The figure shows three views and two pictorial views of one solid part (mm, origin at its lowest corner). Answer the questions. A direction names the side the tool comes from. Coordinates: 2 decimals unless noted, no trailing zeros. Write each loop counter-clockwise with the first axis right and the second up, starting at its lowest first coordinate (ties: lowest second). Pieces come first, ordered by that corner, then holes. Notation, with made-up numbers: M 67.5,53.5 L 92.5,53.5 A12 ccw 92.5,71.5 Z; hole C 26.25,8 d11. An arc over 180 degrees is marked long. Write item = value, one per line.
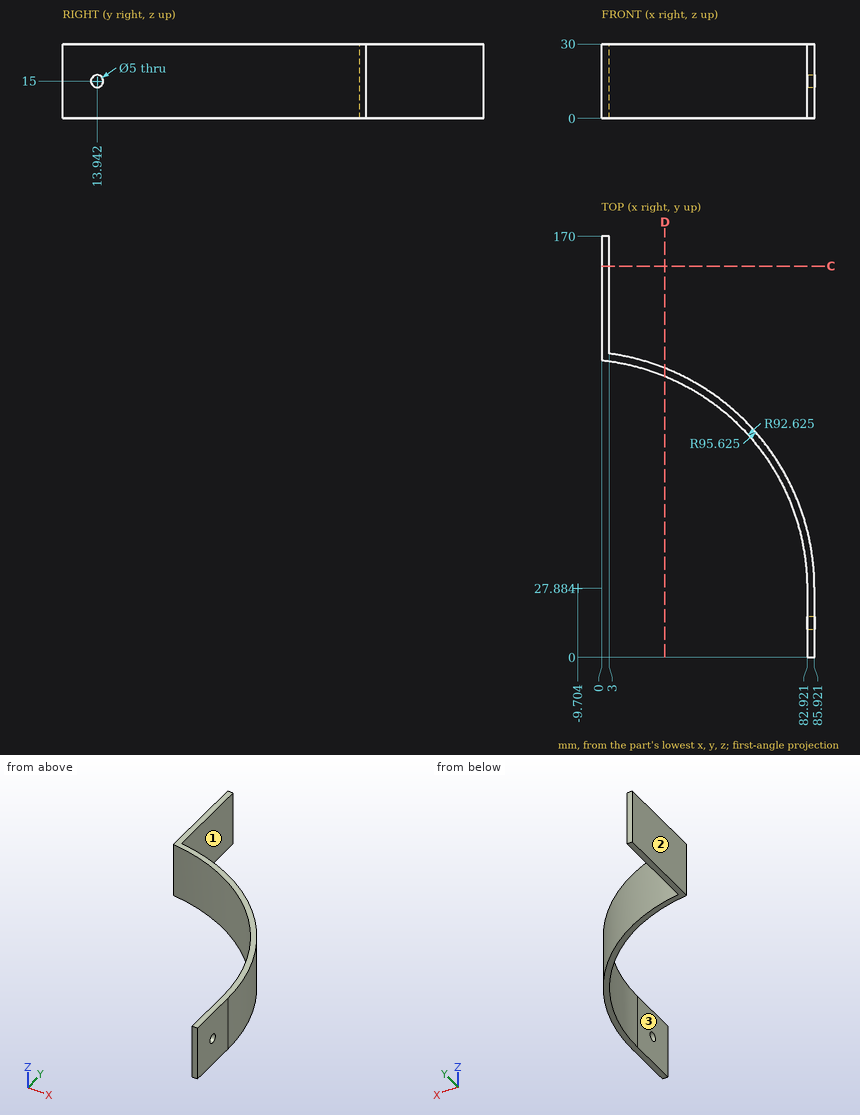
Item 1: Consider line 1 along X through (y, z) = (158, 27.25); line 2 along X through (y, z) = (25, 10); line 3 along Y through (x, z) = (18.5, 13.5) (1 decimal). Determine where each line is inside the solid, lowest interval first. Write a range as from..to.
Worked answers:
line_1 = 0..3
line_2 = 82.92..85.92
line_3 = 116.1..119.3
Item 2: Flat-ended cylindrical pins translate along their axes: pin 1 (10 mm diameter, centred on y = 99, z = 12.5, fed in from +X); pin 2 (14 mm diameter, centred on y = 11, z = 16, fed in from -X); pin 3 (1 mm diameter, centred on y = 56.5, z = 16.5, fed in from +X) (1 decimal). Find the tip coordinate at first contact, or state that the pin passes through.
Worked answers:
pin_1 = 59.38
pin_2 = 82.92
pin_3 = 81.7
Item 3: Find section C-C (y = 158). Determine the outline of the cut face in (x, z).
Worked answers:
outline = M 0,0 L 3,0 L 3,30 L 0,30 Z
Item 4: Find section D-D (x = 25.5). Determine the outline of the cut face in (y, z).
Worked answers:
outline = M 113.56,0 L 116.79,0 L 116.79,30 L 113.56,30 Z
Item 5: Which of the six approach directions +Z, -Z, +X, -X, +Y, -Y give full straight-line access (tool end or side, diameter ignored) to the marked faces 1, 2 and 3?
Worked answers:
face_1 = +Z, -Z, +X, +Y
face_2 = +Z, -Z, -X, +Y, -Y
face_3 = +Z, -Z, -X, -Y
